Geometry check sheet. Reference: the model listing, model coordinates, mm. A direction names the side the tool comes from. Coordinates: 2 decimals unless noted, no trailing zeros. Loops run counter-clockwise (first coordinate to the right, second up) from the corner with the lowest first, then second, coordinate; pieces in that order, holes last.
from build123d import *

# Parameters (mm, degrees)
BOSS_EXTRUDE1_DEPTH = 7.5
BOSS_EXTRUDE2_DEPTH = 22.5
SKETCH1_4_R         = 7.5
BOSS_EXTRUDE3_DEPTH = 14.5


with BuildPart() as part:
    # Sketch1 → Boss-Extrude1 (new, symmetric)
    with BuildSketch(Plane(origin=(0, 0, 0), x_dir=(0, 0, -1), z_dir=(1, 0, 0))):
        with BuildLine():
            ThreePointArc((17.35, 77.82), (0, 95.17), (-17.35, 77.82))
            Line((-17.35, 77.82), (-35, 0))
            Line((-35, 0), (35, 0))
            Line((35, 0), (17.35, 77.82))
        make_face()
    extrude(amount=BOSS_EXTRUDE1_DEPTH, both=True)

    # Sketch1_3 → Boss-Extrude2 (add, symmetric)
    with BuildSketch(Plane(origin=(0, 0, 0), x_dir=(0, 0, -1), z_dir=(1, 0, 0))):
        Polygon((0, 10), (-32.731945515, 10), (-35, 0), (0, 0), align=None)
        Polygon((32.731945515, 10), (0, 10), (0, 0), (35, 0), align=None)
    extrude(amount=BOSS_EXTRUDE2_DEPTH, both=True)

    # Sketch1_4 → Boss-Extrude3 (add)
    with BuildSketch(Plane(origin=(0, 0, 0), x_dir=(0, 0, -1), z_dir=(1, 0, 0))):
        with Locations(Location((0, 77.82, 0), (0, 0, 180))):
            Circle(SKETCH1_4_R)
    extrude(amount=BOSS_EXTRUDE3_DEPTH)


solid = part.part
(1) Draft check along Y on faces 1 (the cylindrical face through (0.105, 95.166, -0.382)), 2 (the flat face through (14.5, 78, 0)), 3 (the flat face through (7.5, 44, 0)). Enter one of: +Y half, -Y half, draft (parallel to the pull), parting line (faces both ways), or undercut.
Findings:
face 1: +Y half
face 2: draft
face 3: undercut
(2) Sectioned sample at B-B on x = -6. Record the cut outline in (y, z), and give its area (3 significant figures).
Findings:
outline: (0, -35) - (77.82, -17.35) arc R17.35 ccw to (77.82, 17.35) - (0, 35) - close
area: 4,550 mm2
(3) Gauge pin test, flat ends, axial feed: pin 1 Ø5 at (y, z) = (77, -14) entering from -X; pin 2 Ø12 at (x, z) = (16, 10) entering from +Y; pin 3 Ø12 at (x, z) = (-15, -2) entering from +Y; pin 4 Ø2 at (x, y) = (17, 77.5) entering from +Z. Record the tip position at first contact, or that the pin passes through.
Findings:
pin 1: stops at x = -7.5
pin 2: stops at y = 84.04
pin 3: stops at y = 10
pin 4: passes through
(4) Scan lines: L1, parallel to X at y = 47.5, z = -18.5; L2, parallel to Y at x = -9.5, z = 7; L3, parallel to Y at x = 1, z = 3. Record each from-to range of solid material in increasing order.
Findings:
L1: x = -7.5 to 7.5
L2: y = 0 to 10
L3: y = 0 to 94.91
(5) Access from +Z, -Z, +X, -X, +Y, -Y to the whole of each face (thin tool, end or side, straight path). Record for faces 4 (the flat face through (0, 0, 0)), 5 (the flat face through (-15, 10, 0)), 6 (the cylindrical face through (10.951, 84.474, 3.461)).
Findings:
face 4: +Z, -Z, +X, -X, -Y
face 5: +Z, -Z, -X, +Y
face 6: +X
(6) Sectioned sample at A-A on z = 0. Record the cut outline in (x, y), and give its area (3 significant figures).
Findings:
outline: (-22.5, 0) - (22.5, 0) - (22.5, 10) - (7.5, 10) - (7.5, 70.32) - (14.5, 70.32) - (14.5, 85.32) - (7.5, 85.32) - (7.5, 95.17) - (-7.5, 95.17) - (-7.5, 10) - (-22.5, 10) - close
area: 1,830 mm2
(7) Sectioned sample at D-D on z = 9. Record the cut outline in (x, y), and give its area (3 significant figures).
Findings:
outline: (-22.5, 0) - (22.5, 0) - (22.5, 10) - (7.5, 10) - (7.5, 92.65) - (-7.5, 92.65) - (-7.5, 10) - (-22.5, 10) - close
area: 1,690 mm2
(8) Sectioned sample at C-C on y = 81. Record the cut outline in (x, z), and give its area (3 significant figures).
Findings:
outline: (-7.5, -17.06) - (7.5, -17.06) - (7.5, -6.79) - (14.5, -6.79) - (14.5, 6.79) - (7.5, 6.79) - (7.5, 17.06) - (-7.5, 17.06) - close
area: 607 mm2
